from build123d import *

# Parameters (mm, degrees)
BOSS_EXTRUDE1_DEPTH     = 10
BOSS_EXTRUDE5_DEPTH     = 5
SKETCH3_W               = 30
SKETCH3_H               = 25
BOSS_EXTRUDE6_DEPTH     = 5
SKETCH4_R               = 3.25
CUT_EXTRUDE1_DEPTH      = 22
CUT_EXTRUDE1_DEPTH_BACK = 17
SKETCH5_R               = 3.25
CUT_EXTRUDE2_DEPTH      = 16
CUT_EXTRUDE2_DEPTH_BACK = 20


with BuildPart() as part:
    # Sketch1 → Boss-Extrude1 (new body)
    with BuildSketch(Plane(origin=(0, 0, 0), x_dir=(0, 0, -1), z_dir=(1, 0, 0))):
        Polygon((0, 0), (-10, 0), (-10, -20), (-30, -20), (-30, -25), (-10, -25), (-10, -47.38), (0, -47.38), align=None)
    extrude(amount=BOSS_EXTRUDE1_DEPTH)

    # Sketch2 → Boss-Extrude5 (add)
    with BuildSketch(Plane.ZY):
        Polygon((0, 0), (10, 0), (10, -20), (30, -20), (30, -25), (0, -25), align=None)
    extrude(amount=BOSS_EXTRUDE5_DEPTH)

    # Sketch3 → Boss-Extrude6 (add)
    with BuildSketch(Plane(origin=(10, 0, 0), x_dir=(0, 0, -1), z_dir=(1, 0, 0))):
        with Locations((-15, -12.5)):
            Rectangle(SKETCH3_W, SKETCH3_H)
    extrude(amount=BOSS_EXTRUDE6_DEPTH)

    # Sketch4 → Cut-Extrude1 (cut, two sides)
    with BuildSketch(Plane(origin=(0, 0, 0), x_dir=(-1, 0, 0), z_dir=(0, 0, -1))) as cut_extrude1_sk:
        with Locations((-1.044087289, -8.964075593)):
            Circle(SKETCH4_R)
    extrude(amount=CUT_EXTRUDE1_DEPTH, mode=Mode.SUBTRACT)
    extrude(cut_extrude1_sk.sketch, amount=-CUT_EXTRUDE1_DEPTH_BACK, mode=Mode.SUBTRACT)

    # Sketch5 → Cut-Extrude2 (cut, two sides)
    with BuildSketch(Plane(origin=(15, 0, 0), x_dir=(0, 0, -1), z_dir=(1, 0, 0))) as cut_extrude2_sk:
        with Locations((-21, -6)):
            Circle(SKETCH5_R)
    extrude(amount=CUT_EXTRUDE2_DEPTH, mode=Mode.SUBTRACT)
    extrude(cut_extrude2_sk.sketch, amount=-CUT_EXTRUDE2_DEPTH_BACK, mode=Mode.SUBTRACT)


solid = part.part
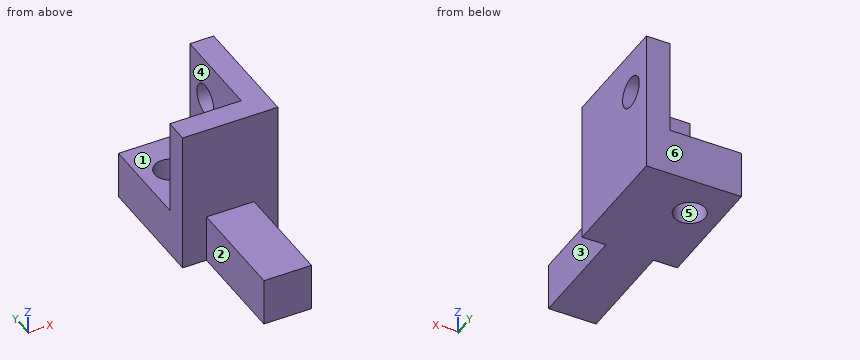
Input: part model. Units: mm. Frame: model coordinates. Face numbers are marked on the shaded views. A direction names the side the tool comes from. Give positions to 0.01 mm unless a question says otherwise; leave off trailing zeros. Write each loop counter-clockwise with the first axis right and the second up, starting at its lowest first coordinate (ties: lowest second). Pieces come first, ordered by that corner, then holes. Notation, with made-up numbers: (-9, 30) -> (47, 30) arc R17 cw to (47, 35) -> close; hole circle Ø8 at (11, -0.75). An arc over 180 degrees is marked (long way). Use one line per item in the form item = value. Start each with the question number.
1) Section query B-B on y = -4. Return the cut outline in (x, z), then the cut area to 3 significant figures.
2) Section query C-C on z = 14.5. Return the cut outline in (x, y), then the cut area to 3 significant figures.
3) Section query A-A on z = 21. Return the cut outline in (x, y), then the cut area to 4 significant figures.
4) Set-up query: the marked faces 1, 2 and 3. Return all of +Z, -Z, +X, -X, +Y, -Y with unobstructed straight access to the full face (end or side cutting, diameter ignored); none if empty.
5) Ray query, probe 1 along Y at (x, z) = (11.4, 21); probe 2 along Y at (x, z) = (-2, 27.25); probe 3 along Z at (x, y) = (1.5, -19.5). Return the intervals inside material, ascending. Write a range as from..to.
6) Draft query along Y for the marked faces 4, 5 and 6. Return one class per face: pulls with the +Y half, pulls with the -Y half, needs draft (parallel to the pull), parting line crosses it, or undercut.
7) Section query D-D on y = -19. Return the cut outline in (x, z).
8) Pin query (flat end, axial travel): pin 1 (6 mm diameter, centred on y = -7, z = 22.5, fed in from -X); pin 2 (8 mm diameter, centred on y = -32.5, z = 4, fed in from -X); pin 3 (11 mm diameter, centred on y = -39, z = 5.5, fed in from +X). Return the tip coordinate at first contact, or that it passes through.
Outcome:
q1.outline = (-5, 0) -> (15, 0) -> (15, 18.44) -> (10, 18.44) -> (10, 10) -> (-5, 10) -> close; (10, 23.56) -> (15, 23.56) -> (15, 30) -> (10, 30) -> close
q1.area = 274 mm^2
q2.outline = (-5, -25) -> (15, -25) -> (15, 0) -> (10, 0) -> (10, -20) -> (-5, -20) -> close
q2.area = 200 mm^2
q3.outline = (-5, -25) -> (15, -25) -> (15, -9.25) -> (10, -9.25) -> (10, -20) -> (-5, -20) -> close; (10, -2.75) -> (15, -2.75) -> (15, 0) -> (10, 0) -> close
q3.area = 167.5 mm^2
q4.face_1 = +Z, -X, +Y
q4.face_2 = +Z, -Z, -X, -Y
q4.face_3 = +Z, -Z, +X, -Y
q5.probe_1 = -25..-9.25, -2.75..0
q5.probe_2 = -25..-20
q5.probe_3 = 0..10
q6.face_4 = needs draft
q6.face_5 = undercut
q6.face_6 = pulls with the +Y half
q7.outline = (-5, 0) -> (15, 0) -> (15, 30) -> (10, 30) -> (10, 10) -> (-5, 10) -> close
q8.pin_1 = 10
q8.pin_2 = 0
q8.pin_3 = 10
